```python
from build123d import *

# Parameters (mm, degrees)
ESQUISSE1_W             = 10
ESQUISSE1_H             = 3.5
BOSS_EXTRU_1_DEPTH      = 2
ENL_V_MAT_EXTRU_1_DEPTH = 29.00542817
BOSS_EXTRU_2_DEPTH      = 3.5
BOSS_EXTRU_3_DEPTH      = 2
ENL_V_MAT_EXTRU_2_REACH = 77.715
ESQUISSE5_R             = 1.3
CONG_1_R                = 3


with BuildPart() as part:
    # Esquisse1 → Boss.-Extru.1 (new body)
    with BuildSketch(Plane.XY):
        with Locations((-66.013415918, -24.332638037)):
            Rectangle(ESQUISSE1_W, ESQUISSE1_H)
    extrude(amount=BOSS_EXTRU_1_DEPTH)

    # Esquisse2 → Enlèv. mat.-Extru.1 (cut, through all)
    with BuildSketch(Plane.ZY.offset(71.013415918)):
        Polygon((2, -25.082638037), (2, -23.582638037), (0.6, -23.232638037), (0.6, -25.432638037), align=None)
    extrude(amount=-ENL_V_MAT_EXTRU_1_DEPTH, mode=Mode.SUBTRACT)

    # Esquisse3 → Boss.-Extru.2 (add)
    with BuildSketch(Plane.XZ.offset(26.082638037)):
        Polygon((-66.513415918, 0), (-66.213415918, -1.1), (-67.813415918, -1.1), (-67.513415918, 0), align=None)
    extrude(amount=-BOSS_EXTRU_2_DEPTH)

    # Esquisse4 → Boss.-Extru.3 (add)
    with BuildSketch(Plane.XY.offset(2)):
        with BuildLine():
            Line((-64.891636129, -22.582638037), (-66.635195707, -22.582638037))
            ThreePointArc((-66.635195707, -22.582638037), (-65.763415918, -18.782638037), (-64.891636129, -22.582638037))
        make_face()
    extrude(amount=-BOSS_EXTRU_3_DEPTH)

    # Esquisse5 → Enlèv. mat.-Extru.2 (cut, up to next)
    with BuildSketch(Plane.XY.offset(2), mode=Mode.PRIVATE) as enl_v_mat_extru_2_sk1:
        with Locations((-65.763415918, -20.782638037)):
            Circle(ESQUISSE5_R)
    enl_v_mat_extru_2_tool1 = extrude(enl_v_mat_extru_2_sk1.sketch, amount=-ENL_V_MAT_EXTRU_2_REACH, mode=Mode.PRIVATE) & part.part
    add(enl_v_mat_extru_2_tool1.solids().sort_by_distance((-65.763416, -20.782638, 2))[0], mode=Mode.SUBTRACT)

    # Congé1
    # the kernel refuses this fillet: 3 mm, written as the material it adds along each edge
    with BuildSketch(Plane(origin=(-66.635195707, -22.582638037, 2), x_dir=(-1, 0, 0), z_dir=(0, 0, -1))) as cong_1_piece_1:
        with BuildLine():
            CenterArc((3.982084651, 3), CONG_1_R, 193.886540363, 76.113459637)
            Line((1.069765987, 2.28), (1.011519614, 2.2656))
            ThreePointArc((1.011519614, 2.2656), (0.884509664, 0.975956702), (-0.026153394, 0.054))
            Line((-0.026153394, 0.054), (0, -0.06))
            Line((0, -0.06), (3.982084651, -0.06))
            Line((3.982084651, -0.06), (3.982084651, 0))
        make_face()
    extrude(amount=2)
    with BuildSketch(Plane(origin=(-64.891636129, -22.582638037, 2), x_dir=(1, 0, 0), z_dir=(0, 0, -1))) as cong_1_piece_2:
        with BuildLine():
            CenterArc((3.982532775, -2.998185933), CONG_1_R, 91.99262488, 74.142247301)
            Line((1.069945237, -2.279274373), (1.011693486, -2.264896142))
            ThreePointArc((1.011693486, -2.264896142), (0.884355653, -0.975628536), (-0.026153394, -0.054))
            Line((-0.026153394, -0.054), (0, 0.06))
            ThreePointArc((0, 0.06), (1.939110106, 0.06), (3.87613396, 0.059963719))
            Line((3.87613396, 0.059963719), (3.878220211, 0))
        make_face()
    extrude(amount=2)


solid = part.part
```
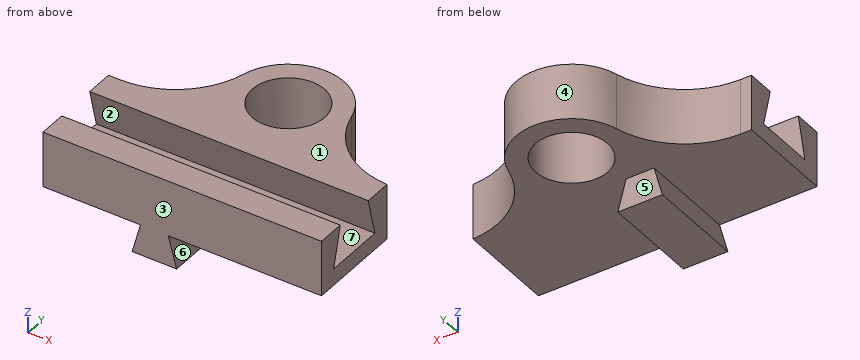
Check sheet for the modelled part. Datum: model origin and axes. Units: mm. Face numbers are marked on the shaded views. A direction names the side the tool comes from. Round coordinates to 2 decimals unless told otherwise and drop trailing zeros. Order: outer loops, then holes, each group sorted by start corner. A loop starts at its lowest first (then second) coordinate and runs counter-clockwise, first axis right, second up.
1) Section check A-A (z = 1.5). Record the boundary of the cut face in (x, y), and give its area (3 significant figures).
2) Mould release check, pull along Z, two halves, no side actions. Record for the marked faces 1, 2 and 3: +Z half, -Z half, draft (parallel to the pull), parting line (faces both ways), or undercut.
3) Go/stop test with a flat-tipped pin: pin 1 Ø1.5 at (x, y) = (-69.5, -24.5) entering from -Z. Record where the tip stops, or that it passes through.
4) Tool access check on the marked faces 4, 5, 6 and 7. Record the directions out of +Z, -Z, +X, -X, +Y, -Y that give a thin tool (end or side, any length) a straight path to the whole face; none if there is none.
5) Section check D-D (y = -23). Record the boundary of the cut face in (x, z), and give its area (3 significant figures).
6) Section check B-B (y = -25.25). Record the boundary of the cut face in (x, z), and give its area (3 significant figures).
7) Section check C-C (x = -66.75). Record the boundary of the cut face in (y, z).
8) Scan lines: line 1 (Z direction, x = -68, y = -25); line 2 (Z direction, x = -64.5, y = -22.25); line 3 (Y direction, x = -62.25, z = 0.7). Record each from-to range of solid material in increasing order.
Result:
1. outline: (-71.01, -26.08) - (-61.01, -26.08) - (-61.01, -25.21) - (-71.01, -25.21) - close; (-71.01, -23.46) - (-61.01, -23.46) - (-61.01, -22.58) arc R3 cw to (-63.82, -20.3) arc R2 ccw to (-67.7, -20.3) arc R3 cw to (-70.62, -22.58) - (-71.01, -22.58) - close; hole circle Ø2.6 at (-65.76, -20.78)
1. area: 28.8 mm2
2. face 1: +Z half
2. face 2: undercut
2. face 3: draft
3. pin 1: stops at z = 0
4. face 4: +Z, -Z, +Y
4. face 5: -Z, +X, -X, +Y
4. face 6: +X, +Y, -Y
4. face 7: +X, -X
5. outline: (-71.01, 0) - (-67.51, 0) - (-67.81, -1.1) - (-66.21, -1.1) - (-66.51, 0) - (-61.01, 0) - (-61.01, 2) - (-71.01, 2) - close
5. area: 21.4 mm2
6. outline: (-71.01, 0) - (-67.51, 0) - (-67.81, -1.1) - (-66.21, -1.1) - (-66.51, 0) - (-61.01, 0) - (-61.01, 0.6) - (-71.01, 0.6) - close; (-71.01, 1.33) - (-61.01, 1.33) - (-61.01, 2) - (-71.01, 2) - close
6. area: 14.1 mm2
7. outline: (-26.08, -1.1) - (-22.58, -1.1) - (-22.58, 0) - (-21.63, 0) - (-21.63, 2) - (-23.58, 2) - (-23.23, 0.6) - (-25.43, 0.6) - (-25.08, 2) - (-26.08, 2) - close; (-19.94, 0) - (-19.04, 0) - (-19.04, 2) - (-19.94, 2) - close
8. line 1: z = 0 to 0.6
8. line 2: z = 0 to 2
8. line 3: y = -26.08 to -25.41, -23.26 to -22.27
